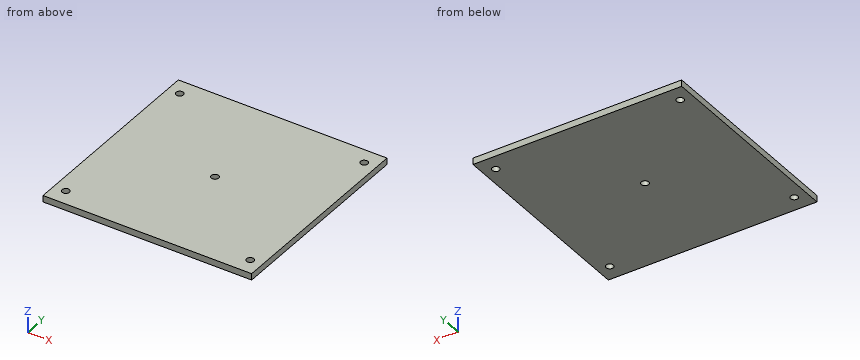
from build123d import *

# Parameters (mm, degrees)
BODY_SKETCH_W    = 97
BODY_SKETCH_H    = 95
BODY_DEPTH       = 3
HOLES_DEPTH      = 136.805007271
HOLES_DEPTH_BACK = 136.805007271
HOLES_SKETCH_R   = 1.7


with BuildPart() as part:
    # Body sketch → Body (new body)
    with BuildSketch(Plane.XY):
        with Locations((48.5, 47.5)):
            Rectangle(BODY_SKETCH_W, BODY_SKETCH_H)
    extrude(amount=BODY_DEPTH)

    # Holes sketch → Holes (cut, two sides: drawn at the far end of the back side and taken through both)
    with BuildSketch(Plane.XY.offset(-HOLES_DEPTH_BACK)):
        with Locations((5.635, 7.495)):
            Circle(HOLES_SKETCH_R)
        with Locations((91.365, 7.495)):
            Circle(HOLES_SKETCH_R)
        with Locations((5.635, 87.505)):
            Circle(HOLES_SKETCH_R)
        with Locations((91.365, 87.505)):
            Circle(HOLES_SKETCH_R)
        with Locations((48.5, 47.5)):
            Circle(HOLES_SKETCH_R)
    extrude(amount=HOLES_DEPTH + HOLES_DEPTH_BACK, mode=Mode.SUBTRACT)


solid = part.part
The model under review builds one solid part; all positions refer to its coordinate system, in mm. Round coordinates to 2 decimals unless told otherwise and drop trailing zeros. Write each loop counter-clockwise with the first axis right and the second up, starting at its lowest first coordinate (ties: lowest second). Pieces come first, ordered by that corner, then holes. Notation, with made-up numbers: (58.25, 34) -> (93.25, 34) arc R28 ccw to (93.25, 52) -> close; hole circle Ø3 at (26.25, 88.25). An arc over 180 degrees is marked (long way). Answer as a JSON object with one key per item and string values.
1. We need section B-B on x = 48.5. State the section outline as (y, z) points.
Results found:
{"outline": "(0, 0) -> (45.8, 0) -> (45.8, 3) -> (0, 3) -> close; (49.2, 0) -> (95, 0) -> (95, 3) -> (49.2, 3) -> close"}
2. To check wall thickness, follow line 1 along Y through (x, z) = (90, 0.2); line 2 along Y through (x, z) = (91, 2.5); line 3 along X through (y, z) = (47.5, 1.65). State the ranges of each line that lie inside material, in increasing order.
Results found:
{"line 1": "y = 0 to 6.48, 8.51 to 86.49, 88.52 to 95", "line 2": "y = 0 to 5.83, 9.16 to 85.84, 89.17 to 95", "line 3": "x = 0 to 46.8, 50.2 to 97"}
3. We need section A-A on y = 47.5. State the section outline as (x, z) points, and give its area (3 significant figures).
Results found:
{"outline": "(0, 0) -> (46.8, 0) -> (46.8, 3) -> (0, 3) -> close; (50.2, 0) -> (97, 0) -> (97, 3) -> (50.2, 3) -> close", "area": "281 mm^2"}
4. Clearance check with flat-ended pins moving along their axes: pin 1 (2.5 mm diameter, centred on x = 5.635, y = 87.505, fed in from +Z); pin 2 (4 mm diameter, centred on x = 91.365, y = 7.495, fed in from -Z). State where each tip first meets the part, or that it passes through.
Results found:
{"pin 1": "passes through", "pin 2": "stops at z = 0"}
